Can you work these out from the model? Positions are in its coordinate system, mm. A direction names the side the tool comes from. Give positions to 0.01 mm unless a question says otherwise; leave off trailing zeros. Loops run counter-clockwise (first coordinate to the right, second up) from the corner with the lowest first, then second, coordinate; pieces in that order, holes last.
from build123d import *

# Parameters (mm, degrees)
SKETCH1_R           = 62.5
SKETCH1_R_2         = 18.25
BOSS_EXTRUDE1_DEPTH = 30
SKETCH2_W           = 16
SKETCH2_H           = 6.75
CUT_EXTRUDE2_DEPTH  = 6
SKETCH3_R           = 43.375
SKETCH3_R_2         = 37.375
CUT_EXTRUDE3_DEPTH  = 10.5
SKETCH5_W           = 7.5
SKETCH5_H           = 4.25
CUT_EXTRUDE5_DEPTH  = 8
CUT_EXTRUDE6_START  = -43.876587737
SKETCH6_R           = 2
CUT_EXTRUDE6_DEPTH  = 53.876587737
CIRPATTERN1_COUNT   = 6
SKETCH7_R           = 2
CUT_EXTRUDE7_DEPTH  = 9.5
CUT_EXTRUDE8_DEPTH  = 4


with BuildPart() as part:
    # Sketch1 → Boss-Extrude1 (new body)
    with BuildSketch(Plane(origin=(0, 0, 0), x_dir=(1, 0, 0), z_dir=(0, 1, 0))):
        Circle(SKETCH1_R)
        Circle(SKETCH1_R_2, mode=Mode.SUBTRACT)
    extrude(amount=BOSS_EXTRUDE1_DEPTH)

    # Sketch2 → Cut-Extrude2 (cut)
    with BuildSketch(Plane(origin=(0, 30, 0), x_dir=(1, 0, 0), z_dir=(0, 1, 0))):
        with Locations((40.375, 0)):
            Rectangle(SKETCH2_W, SKETCH2_H)
        Polygon((19.110335738, -26.350072448), (13.264664262, -29.725072448), (21.264664262, -43.581478908), (27.110335738, -40.206478908), align=None)
        Polygon((-13.264664262, -29.725072448), (-19.110335738, -26.350072448), (-27.110335738, -40.206478908), (-21.264664262, -43.581478908), align=None)
        with Locations((-40.375, 0)):
            Rectangle(SKETCH2_W, SKETCH2_H)
        Polygon((-19.110335738, 26.350072448), (-13.264664262, 29.725072448), (-21.264664262, 43.581478908), (-27.110335738, 40.206478908), align=None)
        Polygon((13.264664262, 29.725072448), (19.110335738, 26.350072448), (27.110335738, 40.206478908), (21.264664262, 43.581478908), align=None)
    extrude(amount=-CUT_EXTRUDE2_DEPTH, mode=Mode.SUBTRACT)

    # Sketch3 → Cut-Extrude3 (cut)
    with BuildSketch(Plane(origin=(0, 30, 0), x_dir=(1, 0, 0), z_dir=(0, 1, 0))):
        Circle(SKETCH3_R)
        Circle(SKETCH3_R_2, mode=Mode.SUBTRACT)
    extrude(amount=-CUT_EXTRUDE3_DEPTH, mode=Mode.SUBTRACT)

    # Sketch5 → Cut-Extrude5 (cut)
    with BuildSketch(Plane(origin=(0, 19.5, 0), x_dir=(1, 0, 0), z_dir=(0, 1, 0))):
        with Locations((0, 40.375)):
            Rectangle(SKETCH5_W, SKETCH5_H)
        Polygon((34.931079661, 24.497595264), (31.250471695, 22.372595264), (35.000471695, 15.877404736), (38.681079661, 18.002404736), align=None)
        Polygon((38.681079661, -18.002404736), (35.000471695, -15.877404736), (31.250471695, -22.372595264), (34.931079661, -24.497595264), align=None)
        with Locations((0, -40.375)):
            Rectangle(SKETCH5_W, SKETCH5_H)
        Polygon((-34.931079661, -24.497595264), (-31.250471695, -22.372595264), (-35.000471695, -15.877404736), (-38.681079661, -18.002404736), align=None)
        Polygon((-38.681079661, 18.002404736), (-35.000471695, 15.877404736), (-31.250471695, 22.372595264), (-34.931079661, 24.497595264), align=None)
    extrude(amount=-CUT_EXTRUDE5_DEPTH, mode=Mode.SUBTRACT)

    # Sketch6 → Cut-Extrude6 (cut)
    with BuildSketch(Plane(origin=(36.806079661, 0, -21.25), x_dir=(0.5, 0, 0.866025404), z_dir=(-0.866025404, 0, 0.5)).offset(CUT_EXTRUDE6_START)):
        with Locations((0, 15.5)):
            Circle(SKETCH6_R)
    cut_extrude6 = extrude(amount=CUT_EXTRUDE6_DEPTH, mode=Mode.SUBTRACT)

    # CirPattern1: Cut-Extrude6 ×6 about axis
    cirpattern1_axis = Axis((0, 0, 0), (0, 1, 0))
    for i in range(1, CIRPATTERN1_COUNT):
        add(cut_extrude6.rotate(cirpattern1_axis, i * 360 / CIRPATTERN1_COUNT), mode=Mode.SUBTRACT)

    # Sketch7 → Cut-Extrude7 (cut)
    with BuildSketch(Plane.XZ):
        with Locations((15.703618414, 51.574778515)):
            Circle(SKETCH7_R)
        with Locations((56.522842607, 7.359909212)):
            Circle(SKETCH7_R)
        with Locations((52.093237989, -15.110557172)):
            Circle(SKETCH7_R)
    extrude(amount=-CUT_EXTRUDE7_DEPTH, mode=Mode.SUBTRACT)

    # Sketch8 → Cut-Extrude8 (cut)
    with BuildSketch(Plane.XZ.offset(-9.5)):
        with BuildLine():
            Line((12.443164797, 54.42424201), (13.733993709, 60.972349609))
            ThreePointArc((13.733993709, 60.972349609), (17.381349368, 60.034479211), (20.965596862, 58.878635754))
            Line((20.965596862, 58.878635754), (19.801552997, 52.973682427))
            Line((19.801552997, 52.973682427), (18.964072031, 48.725315019))
            Line((18.964072031, 48.725315019), (14.866137449, 47.326411107))
            Line((14.866137449, 47.326411107), (11.605683832, 50.175874602))
            Line((11.605683832, 50.175874602), (12.443164797, 54.42424201))
        make_face()
        with BuildLine():
            Line((54.942701485, -11.850103555), (50.694334077, -11.012622589))
            Line((50.694334077, -11.012622589), (47.844870581, -14.273076206))
            Line((47.844870581, -14.273076206), (49.243774494, -18.371010788))
            Line((49.243774494, -18.371010788), (53.492141902, -19.208491754))
            Line((53.492141902, -19.208491754), (59.106200943, -20.315191608))
            ThreePointArc((59.106200943, -20.315191608), (60.22155233, -16.721681583), (61.118644269, -13.06756759))
            Line((61.118644269, -13.06756759), (54.942701485, -11.850103555))
        make_face()
        with BuildLine():
            Line((59.372306103, 10.620362829), (55.123938695, 11.457843794))
            Line((55.123938695, 11.457843794), (52.274475199, 8.197390178))
            Line((52.274475199, 8.197390178), (53.673379112, 4.099455595))
            Line((53.673379112, 4.099455595), (57.92174652, 3.261974629))
            Line((57.92174652, 3.261974629), (62.455112673, 2.368311841))
            ThreePointArc((62.455112673, 2.368311841), (62.183643054, 6.280488561), (61.667357766, 10.167939133))
            Line((61.667357766, 10.167939133), (59.372306103, 10.620362829))
        make_face()
    extrude(amount=CUT_EXTRUDE8_DEPTH, mode=Mode.SUBTRACT)


solid = part.part
(1) Please list where these lines run through material, in increasing order: probe 1 along Z at (x, y) = (0, 21.25) (3 decimals); probe 2 along Z at (x, y) = (-2.5, 17); probe 3 along Z at (x, y) = (0, 7).
Returned:
probe 1: z = -62.5 to -43.375, -37.375 to -18.25, 18.25 to 37.375, 43.375 to 62.5
probe 2: z = -62.45 to -42.5, -38.25 to -18.08, 18.08 to 38.25, 42.5 to 62.45
probe 3: z = -62.5 to -18.25, 18.25 to 62.5
(2) Suppose I cut it at A-A on z = 0. List the corners of the cut face in (x, y) for me (3 decimals).
Returned:
outline: (-62.5, 0) - (-18.25, 0) - (-18.25, 30) - (-32.375, 30) - (-32.375, 24) - (-37.375, 24) - (-37.375, 19.5) - (-43.375, 19.5) - (-43.375, 24) - (-48.375, 24) - (-48.375, 30) - (-62.5, 30) - close; (18.25, 0) - (62.5, 0) - (62.5, 30) - (48.375, 30) - (48.375, 24) - (43.375, 24) - (43.375, 19.5) - (37.375, 19.5) - (37.375, 24) - (32.375, 24) - (32.375, 30) - (18.25, 30) - close
(3) Thinking about a two-plate mould opening in Z: for faces 3 (the flat face through (0, 11.5, 40)), 4 (the flat face through (0, 16, -32.5)), 5 (the flat face through (13.014, 0, 13.014)), which applies, pulls with the +Z half, pulls with the -Z half, needs draft (parallel to the pull), parting line crosses it, or undercut?
Returned:
face 3: undercut
face 4: pulls with the -Z half
face 5: needs draft
(4) Suppose I cut it at D-D on y = 22.5. List the corners of the cut face in (x, z) for me (3 decimals), plus the area to 3 significant figures.
Returned:
outline: circle Ø125 at (0, 0); circle Ø74.75 at (0, 0); hole circle Ø86.75 at (0, 0); hole circle Ø36.5 at (0, 0)
area: 9,700 mm2
(5) Suppose I cut it at B-B on y = 7. List the corners of the cut face in (x, z) for me, plus the area to 3 significant figures.
Returned:
outline: (11.61, 50.18) - (13.73, 60.97) arc R62.5 ccw (long way) to (59.11, -20.32) - (49.24, -18.37) - (47.84, -14.27) - (50.69, -11.01) - (61.12, -13.07) arc R62.5 ccw to (62.46, 2.37) - (53.67, 4.1) - (52.27, 8.2) - (55.12, 11.46) - (61.67, 10.17) arc R62.5 ccw to (20.97, 58.88) - (18.96, 48.73) - (14.87, 47.33) - close; hole circle Ø36.5 at (0, 0)
area: 11,000 mm2
(6) Will these pins go through, and if not, where does the flat tip stop? P1, Ø2.5, axis at x = 46.5, y = 27, coming from the -Z side; P2, Ø1, axis at y = 15.5, z = -45.5, coming from the +X side; P3, Ø4, axis at x = -18, y = 15, coming from the +Z side.
Returned:
P1: stops at z = -43.11
P2: stops at x = 43.37
P3: stops at z = 60.42
(7) Which directions (+Z, -Z, +X, -X, +Y, -Y) give clear straight access to the entire face, cutting with the end or side of a thin tool? Please do faces 1 (the flat face through (54.4, 5.5, -15.6)), 2 (the flat face through (-16, 19.5, 35)).
Returned:
face 1: none
face 2: +Y
(8) Suppose I cut it at C-C on x = -11. List the corners of the cut face in (y, z) for me.
Returned:
outline: (0, -61.52) - (30, -61.52) - (30, -41.96) - (19.5, -41.96) - (19.5, -35.72) - (30, -35.72) - (30, -14.56) - (0, -14.56) - close; (0, 14.56) - (30, 14.56) - (30, 35.72) - (19.5, 35.72) - (19.5, 41.96) - (30, 41.96) - (30, 61.52) - (0, 61.52) - close
